```python
from build123d import *

# Parameters (mm, degrees)
SKETCH1_W           = 82.55
SKETCH1_H           = 292.1
BOSS_EXTRUDE1_DEPTH = 3.175
CUT_EXTRUDE1_REACH  = 305.557
SKETCH2_W           = 50.25
SKETCH2_H           = 19.5
CUT_EXTRUDE2_REACH  = 305.557
SKETCH4_R           = 10.25
CUT_EXTRUDE3_REACH  = 305.557
SKETCH5_W           = 13.7
SKETCH5_H           = 8.55
CUT_EXTRUDE4_REACH  = 305.557
SKETCH6_R           = 12.25
SKETCH6_R_2         = 10.25
SKETCH6_W           = 54.25
SKETCH6_H           = 23.5
SKETCH6_W_2         = 50.25
SKETCH6_H_2         = 19.5
SKETCH6_W_3         = 17.7
SKETCH6_H_3         = 12.55
SKETCH6_W_4         = 13.7
SKETCH6_H_4         = 8.55
SKETCH7_W           = 3.175
SKETCH7_H           = 292.1
BOSS_EXTRUDE2_DEPTH = 3.175


with BuildPart() as part:
    # Sketch1 → Boss-Extrude1 (new body)
    with BuildSketch(Plane(origin=(0, 0, 0), x_dir=(0, 0, -1), z_dir=(1, 0, 0))):
        with Locations((41.275, 146.05)):
            Rectangle(SKETCH1_W, SKETCH1_H)
    extrude(amount=BOSS_EXTRUDE1_DEPTH)

    # Sketch2 → Cut-Extrude1 (cut, up to next)
    with BuildSketch(Plane.ZY, mode=Mode.PRIVATE) as cut_extrude1_sk1:
        with Locations((-41.275, 244.25)):
            Rectangle(SKETCH2_W, SKETCH2_H)
    cut_extrude1_tool1 = extrude(cut_extrude1_sk1.sketch, amount=-CUT_EXTRUDE1_REACH, mode=Mode.PRIVATE) & part.part
    add(cut_extrude1_tool1.solids().sort_by_distance((0, 244.25, -41.275))[0], mode=Mode.SUBTRACT)

    # Sketch4 → Cut-Extrude2 (cut, up to next)
    with BuildSketch(Plane.ZY, mode=Mode.PRIVATE) as cut_extrude2_sk1:
        with Locations((-41.275, 127)):
            Circle(SKETCH4_R)
    cut_extrude2_tool1 = extrude(cut_extrude2_sk1.sketch, amount=-CUT_EXTRUDE2_REACH, mode=Mode.PRIVATE) & part.part
    add(cut_extrude2_tool1.solids().sort_by_distance((0, 127, -41.275))[0], mode=Mode.SUBTRACT)

    # Sketch5 → Cut-Extrude3 (cut, up to next)
    with BuildSketch(Plane.ZY, mode=Mode.PRIVATE) as cut_extrude3_sk1:
        with Locations((-41.275, 29.675)):
            Rectangle(SKETCH5_W, SKETCH5_H)
    cut_extrude3_tool1 = extrude(cut_extrude3_sk1.sketch, amount=-CUT_EXTRUDE3_REACH, mode=Mode.PRIVATE) & part.part
    add(cut_extrude3_tool1.solids().sort_by_distance((0, 29.675, -41.275))[0], mode=Mode.SUBTRACT)

    # Sketch6 → Cut-Extrude4 (cut, up to next)
    with BuildSketch(Plane.ZY, mode=Mode.PRIVATE) as cut_extrude4_sk1:
        with Locations((-41.275, 127)):
            Circle(SKETCH6_R)
        with Locations((-41.275, 127)):
            Circle(SKETCH6_R_2, mode=Mode.SUBTRACT)
    cut_extrude4_tool1 = extrude(cut_extrude4_sk1.sketch, amount=-CUT_EXTRUDE4_REACH, mode=Mode.PRIVATE) & part.part
    # Sketch6 → Cut-Extrude4 (cut, up to next)
    with BuildSketch(Plane.ZY, mode=Mode.PRIVATE) as cut_extrude4_sk2:
        with Locations((-41.275, 244.25)):
            Rectangle(SKETCH6_W, SKETCH6_H)
        with Locations((-41.275, 244.25)):
            Rectangle(SKETCH6_W_2, SKETCH6_H_2, mode=Mode.SUBTRACT)
    cut_extrude4_tool2 = extrude(cut_extrude4_sk2.sketch, amount=-CUT_EXTRUDE4_REACH, mode=Mode.PRIVATE) & part.part
    # Sketch6 → Cut-Extrude4 (cut, up to next)
    with BuildSketch(Plane.ZY, mode=Mode.PRIVATE) as cut_extrude4_sk3:
        with Locations((-41.275, 29.675)):
            Rectangle(SKETCH6_W_3, SKETCH6_H_3)
        with Locations((-41.275, 29.675)):
            Rectangle(SKETCH6_W_4, SKETCH6_H_4, mode=Mode.SUBTRACT)
    cut_extrude4_tool3 = extrude(cut_extrude4_sk3.sketch, amount=-CUT_EXTRUDE4_REACH, mode=Mode.PRIVATE) & part.part
    add(cut_extrude4_tool1.solids().sort_by_distance((0, 127, -53.178518))[0], mode=Mode.SUBTRACT)
    add(cut_extrude4_tool2.solids().sort_by_distance((0, 255.408788, -41.275))[0], mode=Mode.SUBTRACT)
    add(cut_extrude4_tool3.solids().sort_by_distance((0, 35.733022, -41.275))[0], mode=Mode.SUBTRACT)


with BuildPart() as body_2:
    # Sketch7 → Boss-Extrude2 (new body)
    with BuildSketch(Plane(origin=(3.175, 0, 0), x_dir=(0, 0, -1), z_dir=(1, 0, 0))):
        with Locations((-1.5875, 146.05)):
            Rectangle(SKETCH7_W, SKETCH7_H)
    extrude(amount=-BOSS_EXTRUDE2_DEPTH)


with BuildPart() as part_1:
    add(part.part)

    # Combine1: union body 2
    add(body_2.part)


solid = part_1.part
```
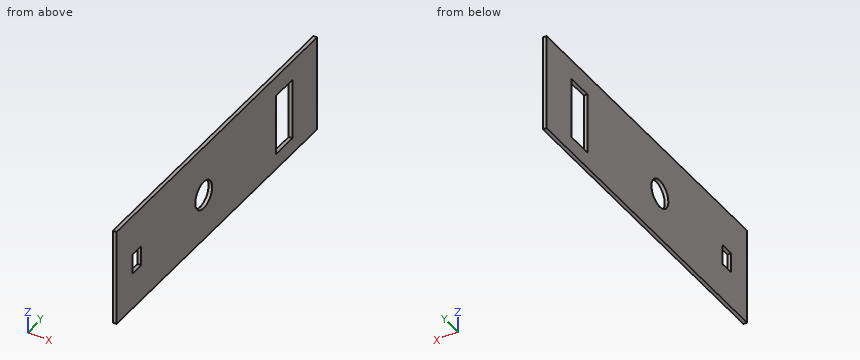
Could you check a few things on this model? Use its own coordinates, in mm. Round coordinates to 2 decimals unless told otherwise and drop trailing zeros. Loops run counter-clockwise (first coordinate to the right, second up) from the corner with the lowest first, then second, coordinate; pieces in that order, holes last. Notation, with made-up numbers: M 86,-20.75 L 133,-20.75 A13 ccw 133,-3.75 Z; hole C 55.5,77 d6. An arc over 180 degrees is marked long. Put each result on its own line as item: value.
Q1. Imagine slicing it at B-B (z = -56). Write out the boundary of the cut face in (x, y) (3 decimals), then the cut area to 3 significant figures.
Check result:
outline: M 0,0 L 3.175,0 L 3.175,232.5 L 0,232.5 Z; M 0,256 L 3.175,256 L 3.175,292.1 L 0,292.1 Z
area: 853 mm2
Q2. Imagine slicing it at A-A (y = 127). Write out the boundary of the cut face in (x, z) (3 decimals), then the cut area to 3 significant figures.
Check result:
outline: M 0,-82.55 L 3.175,-82.55 L 3.175,-53.525 L 0,-53.525 Z; M 0,-29.025 L 3.175,-29.025 L 3.175,3.175 L 0,3.175 Z
area: 194 mm2
Q3. Imagine slicing it at C-C (x = 1.65). Write out the boundary of the cut face in (y, z) (3 decimals), then the cut area to 3 significant figures.
Check result:
outline: M 0,-82.55 L 292.1,-82.55 L 292.1,3.175 L 0,3.175 Z; hole M 23.4,-50.125 L 35.95,-50.125 L 35.95,-32.425 L 23.4,-32.425 Z; hole C 127,-41.275 d24.5; hole M 232.5,-68.4 L 256,-68.4 L 256,-14.15 L 232.5,-14.15 Z
area: 23,100 mm2
Q4. For pin 1 (14.5 mm diameter, centred on y = 127, z = -41.275, fed in from +X), with a flat end and sliding along its axis, tell me the tip position at first contact or that it passes through.
Check result:
pin 1: through
Q5. I need wall thicknesses on probe 1 along Y at (x, z) = (2.25, -41); probe 2 along Y at (x, z) = (0.75, -50.5); probe 3 along Y at (x, z) = (0.5, -68). Which ranges of each line are inside material? Lowest first, please.
Check result:
probe 1: 0 to 23.4, 35.95 to 114.75, 139.25 to 232.5, 256 to 292.1
probe 2: 0 to 118.94, 135.06 to 232.5, 256 to 292.1
probe 3: 0 to 232.5, 256 to 292.1
